The model under review builds one solid part; all positions refer to its coordinate system, in mm. Face numbers are marked on the shaded views. A direction names the side the tool comes from. Round coordinates to 2 decimals unless told otherwise and drop trailing zeros. Loops run counter-clockwise (first coordinate to the right, second up) from the corner with the lowest first, then second, coordinate; pieces in that order, holes last. Notation, with made-up numbers: M -14.5,27.25 L 11.5,27.25 A10 ccw 11.5,35.25 Z; hole C -33.75,-15.5 d1. An arc over 180 degrees is marked long. Use a Markdown table: item, result. Add a question column.
Autodesk Inventor part; units mm, degrees
ref_plane "YZ Plane" through (0, 0, 0) normal (1, 0, 0) x (0, 1, 0)
ref_plane "XZ Plane" through (0, 0, 0) normal (0, 1, 0) x (-1, 0, 0)
ref_plane "XY Plane" through (0, 0, 0) normal (0, 0, 1) x (1, 0, 0)
sketch "Sketch1" plane through (0, 0, 0) normal (0, 0, 1) x (1, 0, 0)
  line L0 (-2.5718, -2.6632) -> (-7.5718, -2.6632)
  line L1 (-7.5718, -2.6632) -> (-7.5718, -80.8132)
  line L2 (-7.5718, -80.8132) -> (-2.5718, -80.8132)
  line L3 (-2.5718, -80.8132) -> (-2.5718, -2.6632)
  dimension "d1" = 78.15
  dimension "d2" = 5
revolve "Shoulder" add sketch "Sketch1" angle 360 about axis through (-2.5718, -80.8132, 0) along (0, 1, 0)
sketch "Sketch2" plane through (-2.5718, -2.6632, 0) normal (0, 1, 0) x (1, 0, 0)
  circle A0 centre (0, 0) radius 5
  circle A1 centre (0, 0) radius 4.76
  dimension "d3" = 9.52
extrude "Shoulder_neck" add sketch "Sketch2" along normal blind 1.85 contours A1
sketch "Sketch3" plane through (-2.5718, -0.8132, 0) normal (0, 1, 0) x (1, 0, 0)
  circle A0 centre (0, 0) radius 4.76
  circle A1 centre (0, 0) radius 8.1
  dimension "d6" = 16.2
extrude "Head" add sketch "Sketch3" along normal blind 7 contours A0 | A1
sketch "Sketch4" plane through (-2.5718, -80.8132, 0) normal (0, -1, 0) x (1, 0, 0)
  circle A0 centre (0, 0) radius 5
  circle A1 centre (0, 0) radius 3.09
  dimension "d9" = 6.18
extrude "Thread_neck" add sketch "Sketch4" along normal blind 2.6 contours A1
sketch "Sketch5" plane through (-2.5718, -83.4132, 0) normal (0, -1, 0) x (1, 0, 0)
  circle A0 centre (0, 0) radius 3.09
  circle A1 centre (0, 0) radius 4
  dimension "d12" = 8
extrude "Thread_shoulder" add sketch "Sketch5" along normal blind 10.4 contours A0 | A1
sketch "Sketch6" plane through (-2.5718, 6.1868, 0) normal (0, 1, 0) x (1, 0, 0)
  circle A0 centre (0, 0) radius 8.1
  circle A1 centre (0, 0) radius 2.5 construction
  line L0 (-2.5, 1.4434) -> (-2.5, -1.4434)
  line L1 (-2.5, -1.4434) -> (0, -2.8868)
  line L2 (0, -2.8868) -> (2.5, -1.4434)
  line L3 (2.5, -1.4434) -> (2.5, 1.4434)
  line L4 (2.5, 1.4434) -> (0, 2.8868)
  line L5 (0, 2.8868) -> (-2.5, 1.4434)
  dimension "d15" = 5
extrude "Hex" cut sketch "Sketch6" against normal blind 4.2 contours L5 L4 L3 L2 L1 L0
chamfer "Chamfer1" distance 0.24 angle 30 1 edges at (2.4282, -2.6632, 0) measured on face at (-7.3973, -2.6632, -0.7786)
fillet "Fillet1" radius 0.4 1 edges at (-7.3318, -0.8132, 0)
chamfer "Chamfer2" distance 0.5 angle 30 1 edges at (-10.6718, 6.1868, 0) measured on face at (5.4233, 3.8535, 1.2993)
chamfer "Chamfer3" distance 0.625 angle 30 1 edges at (-6.5718, -93.8132, 0) measured on face at (-1.8144, -93.8132, 1.0973)
fillet "Fillet2" radius 0.7 1 edges at (-5.6618, -80.8132, 0)
chamfer "Chamfer7" distance 0.91 angle 30 1 edges at (-6.5718, -83.4132, 0) measured on face at (1.0861, -83.4132, -0.3191)
thread "Thread"
equation "\"d1\" = Shoulder_length - Shoulder_neck_length"
equation "\"d2\" = 0.5 * Shoulder_diameter"
equation "\"d3\" = Shoulder_neck_dia"
equation "\"d4\" = Shoulder_neck_length"
equation "\"d6\" = Head_diameter"
equation "\"d7\" = Head_height"
equation "\"d9\" = Thread_neck_dia"
equation "\"d10\" = Thread_neck_length"
equation "\"d12\" = Thread_diameter"
equation "\"d13\" = Thread_length - Thread_neck_length"
equation "\"d15\" = Hex_size"
equation "\"d16\" = Hex_length"
equation "\"d18\" = -0.5 * Shoulder_neck_dia + 0.5 * Shoulder_diameter"
equation "\"d64\" = -0.5 * Shoulder_neck_dia + 0.5 * Shoulder_diameter"
equation "\"d21\" = 0.1 * Hex_size"
equation "\"d65\" = 0.1 * Hex_size"
equation "\"d23\" = 0.5 * Thread_pitch"
equation "\"d66\" = 0.5 * Thread_pitch"
equation "\"d25\" = Thread_neck_radius"
equation "\"d60\" = -0.5 * Thread_neck_dia + 0.5 * Thread_diameter"
equation "\"d67\" = -0.5 * Thread_neck_dia + 0.5 * Thread_diameter"
equation "\"Shoulder_length\" = 80"
equation "\"Shoulder_neck_dia\" = 9.52"
equation "\"Thread_diameter\" = 8"
equation "\"Thread_length\" = 13"
equation "\"Head_diameter\" = 16.2"
equation "\"Head_height\" = 7"
equation "\"Thread_neck_dia\" = 6.18"
equation "\"Hex_size\" = 5"
equation "\"Hex_length\" = 4.2"
equation "\"Thread_pitch\" = 1.25"
equation "\"Shoulder_neck_length\" = 1.85"
equation "\"Thread_neck_length\" = 2.6"
equation "\"Thread_neck_radius\" = 0.7"
properties part number "SCREW, SHOULDER, P, 12.9,  M10X80MM" material "Steel, High Strength Low Alloy"
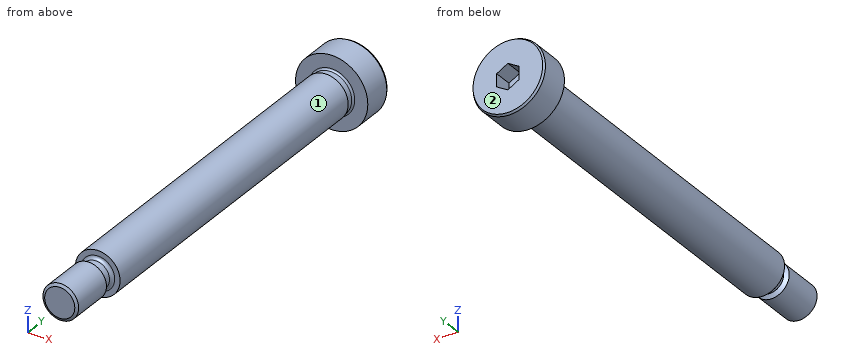
(1) Consider section A-A, the plane y = -55.5. Give the boundary of the cut face in (x, z).
(2) To check wall thickness, follow probe 1 along Y at (x, z) = (3.5, -0.25); probe 2 along Y at (x, z) = (-4.75, -0.75); probe 3 along X at (y, z) = (-73.5, 1.5). State the ranges of each line that lie inside material, in increasing order.
(3) Insertion check: pin 1 Ø1.5 at (x, y) = (-6.5, -60.5) entering from +Z; pin 2 Ø8 at (y, z) = (-25, -5) entering from -X; pin 3 Ø6 at (y, z) = (-77, 0.5) entering from -X. Each pin has a flat end and moves straight along its axis. Give the tip position at first contact, or say it passes through.
(4) For the marked faces 1 and 2, list the 3-axis set-ups (+Z, -Z, +X, -X, +Y, -Y) from which the entire face can be reached by the end or side of a thin tool; tool diameter is ignored.
Found:
| question | item | result |
|---|---|---|
| 1 | outline | C -2.57,0 d10 |
| 2 | probe 1 | y = -0.81 to 6.19 |
| 2 | probe 2 | y = -93.81 to 1.99 |
| 2 | probe 3 | x = -7.34 to 2.2 |
| 3 | pin 1 | stops at z = 3.86 |
| 3 | pin 2 | stops at x = -7.47 |
| 3 | pin 3 | stops at x = -7.57 |
| 4 | face 1 | -Y |
| 4 | face 2 | +Z, -Z, +X, -X, +Y |
